Read the model definition and answer for the solid it produces. Units are mm, in the model's axes. Coordinates: 2 decimals unless noted, no trailing zeros. Write each loop counter-clockwise with the first axis right and the second up, starting at its lowest first coordinate (ties: lowest second). Pieces come first, ordered by that corner, then holes. Notation, with made-up numbers: (26.5, 64.5) -> (54.5, 64.5) arc R13 ccw to (54.5, 89.5) -> close; hole circle Ø7 at (14, 56). An arc over 180 degrees is marked (long way). Return JSON: item names as keys, results as strings.
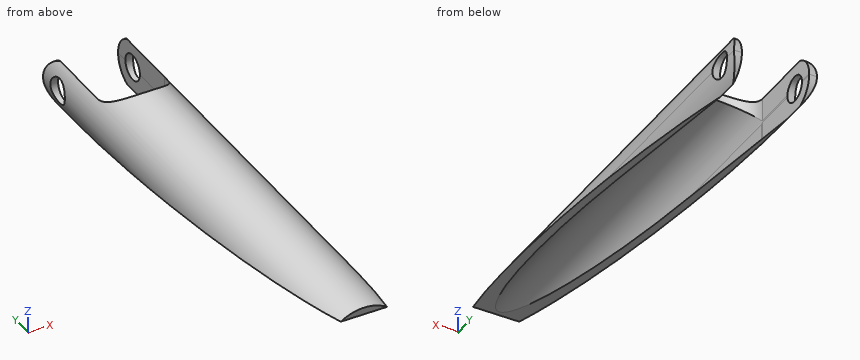
from build123d import *

# Parameters (mm, degrees)
F0_R          = 12.7
F0_R_2        = 10.31875
F1_DEPTH      = 152.4
F2_R          = 3.96875
F3_DEPTH      = 25.4
F3_DEPTH_BACK = 25.4
F5_DEPTH      = 12.7
F7_DEPTH      = 12.7
F8_W          = 20.6375
F8_H          = 12.7
F9_DEPTH      = 127
F11_DEPTH     = 12.7


with BuildPart() as f1:
    # F0 (on Front) → F1 (new body)
    with BuildSketch(Plane.XZ):
        Circle(F0_R)
        Circle(F0_R_2, mode=Mode.SUBTRACT)
    extrude(amount=F1_DEPTH)

    # F2 (on Right) → F3 (cut, two sides)
    with BuildSketch(Plane.YZ) as f3_sk:
        with Locations((-7.9375, 0)):
            Circle(F2_R)
    extrude(amount=F3_DEPTH, mode=Mode.SUBTRACT)
    extrude(f3_sk.sketch, amount=-F3_DEPTH_BACK, mode=Mode.SUBTRACT)

    # F4 (on Top) → F5 (cut, symmetric)
    with BuildSketch(Plane.XY):
        with BuildLine():
            Line((-10.315392, 0), (-10.315392, -25.4))
            ThreePointArc((-10.315392, -25.4), (0.001679, -35.717071), (10.31875, -25.4))
            Line((10.31875, -25.4), (10.31875, 0))
            Line((10.31875, 0), (-10.315392, 0))
        make_face()
    extrude(amount=F5_DEPTH, both=True, mode=Mode.SUBTRACT)

    # F6 (on Right) → F7 (cut, symmetric)
    with BuildSketch(Plane.YZ):
        Polygon((-11.90625, -7.313158), (-152.4, 10.53286), (-152.4, -12.869733), (-11.961568, -12.869733), align=None)
    extrude(amount=F7_DEPTH, both=True, mode=Mode.SUBTRACT)

    # F8 (on Front) → F9 (cut)
    with BuildSketch(Plane.XZ):
        with Locations((0.022642, -6.35)):
            Rectangle(F8_W, F8_H)
    extrude(amount=F9_DEPTH, mode=Mode.SUBTRACT)

    # F10 (on Right) → F11 (cut, symmetric)
    with BuildSketch(Plane.YZ):
        with BuildLine():
            ThreePointArc((-7.9375, 7.9375), (-2.32484, 5.61266), (0, 0))
            Line((0, 0), (0, 7.9375))
            Line((0, 7.9375), (-7.9375, 7.9375))
        make_face()
        with BuildLine():
            ThreePointArc((0, 0), (-2.32484, -5.61266), (-7.9375, -7.9375))
            Line((-7.9375, -7.9375), (0, -7.9375))
            Line((0, -7.9375), (0, 0))
        make_face()
    extrude(amount=F11_DEPTH, both=True, mode=Mode.SUBTRACT)


solid = f1.part
1. The part is cut by section B-B (z = 5.25). Determine the outline of the cut face in (x, y).
Taken from the geometry:
{"outline": "(-11.56, -110.81) -> (-8.88, -110.81) -> (-8.88, -30.64) arc R10.32 cw to (-10.32, -25.4) -> (-10.32, -1.98) -> (-11.56, -1.98) -> close; (8.88, -110.81) -> (11.56, -110.81) -> (11.56, -1.98) -> (10.32, -1.98) -> (10.32, -25.4) arc R10.32 cw to (8.88, -30.65) -> close"}
2. The part is cut by section C-C (y = -10.5). Determine the outline of the cut face in (x, z).
Taken from the geometry:
{"outline": "(-12.33, -3.03) arc R12.7 ccw to (-10.32, -7.41) -> (-10.32, -3.03) -> close; (-12.33, 3.03) -> (-10.32, 3.03) -> (-10.32, 7.41) arc R12.7 ccw to start; (10.32, 3.03) -> (12.33, 3.03) arc R12.7 ccw to (10.32, 7.4) -> close; (10.34, -7.37) arc R12.7 ccw to (12.33, -3.03) -> (10.34, -3.03) -> close"}
3. Consider L1, parallel to X at y = -15.5, z = -3.25; L2, parallel to X at y = -38, z = 0.5; L3, parallel to Z at x = 6, y = -97. Determine where each line is inside the solid, lowest interval first.
Taken from the geometry:
{"L1": "x = -12.28 to -10.32, 10.34 to 12.28", "L2": "x = -12.69 to -10.31, 10.31 to 12.69", "L3": "z = 8.4 to 11.19"}
4. The part is cut by section D-D (x = 0). Determine the outline of the cut face in (y, z).
Taken from the geometry:
{"outline": "(-152.4, 10.53) -> (-150.71, 10.32) -> (-35.72, 10.32) -> (-35.72, 12.7) -> (-152.4, 12.7) -> close"}
5. Flat-ended cylindrical pins translate along their axes: pin 1 Ø1.5 at (y, z) = (-104, 2) entering from -X; pin 2 Ø10 at (x, z) = (6, 8.5) entering from +Y; pin 3 Ø3.5 at (y, z) = (-18, 2) entering from +X; pin 4 Ø12 at (x, z) = (-2.5, 6.5) entering from +Y. Find the tip coordinate at first contact, or state that the pin passes through.
Taken from the geometry:
{"pin 1": "passes through", "pin 2": "stops at y = -2.72", "pin 3": "stops at x = 12.7", "pin 4": "stops at y = -31.24"}
